```python
from build123d import *

# Parameters (mm, degrees)
SKETCH1_R           = 82.5
BOSS_EXTRUDE1_DEPTH = 17
SKETCH2_R           = 40
CUT_EXTRUDE1_DEPTH  = 118.904622471
SKETCH3_R           = 5.652492576
CUT_EXTRUDE2_DEPTH  = 12.839244
CIRPATTERN1_START   = 4.160755595
CIRPATTERN1_DEPTH   = 12.839244405


# Read off the part's stored shape, not the designer's step: CirPattern1
with BuildPart() as part:
    # Sketch1 → Boss-Extrude1 (new body)
    with BuildSketch(Plane(origin=(0, 0, 0), x_dir=(1, 0, 0), z_dir=(0, 1, 0))):
        with Locations(Location((0, 0, 0), (0, 0, 270))):
            Circle(SKETCH1_R)
    extrude(amount=BOSS_EXTRUDE1_DEPTH)

    # Sketch2 → Cut-Extrude1 (cut, through all)
    with BuildSketch(Plane(origin=(0, 0, 0), x_dir=(1, 0, 0), z_dir=(0, 1, 0))):
        with Locations(Location((0, 0, 0), (0, 0, 270))):
            Circle(SKETCH2_R)
    extrude(amount=CUT_EXTRUDE1_DEPTH, mode=Mode.SUBTRACT)

    # Sketch3 → Cut-Extrude2 (cut)
    with BuildSketch(Plane(origin=(0, 17, 0), x_dir=(1, 0, 0), z_dir=(0, 1, 0))):
        with Locations((-36.098285333, 0)):
            Circle(SKETCH3_R)
    extrude(amount=-CUT_EXTRUDE2_DEPTH, mode=Mode.SUBTRACT)

    # CirPattern1 outline → CirPattern1 (cut)
    with BuildSketch(Plane(origin=(0, 0, 0), x_dir=(1, 0, 0), z_dir=(0, 1, 0)).offset(CIRPATTERN1_START)):
        with BuildLine():
            ThreePointArc((-4.299022975, 39.768309009), (0, 40), (4.299022975, 39.768309009))
            ThreePointArc((4.299022975, 39.768309009), (0, 41.75077791), (-4.299022975, 39.768309009))
        make_face()
        with BuildLine():
            ThreePointArc((39.768309009, -4.299022975), (41.75077791, 0), (39.768309009, 4.299022975))
            ThreePointArc((39.768309009, 4.299022975), (40, 0), (39.768309009, -4.299022975))
        make_face()
        with BuildLine():
            ThreePointArc((4.299022975, -39.768309009), (0, -40), (-4.299022975, -39.768309009))
            ThreePointArc((-4.299022975, -39.768309009), (0, -41.75077791), (4.299022975, -39.768309009))
        make_face()
    extrude(amount=CIRPATTERN1_DEPTH, mode=Mode.SUBTRACT)


solid = part.part
```
Design review of the part built by this model. Coordinates are the model's own, in mm. A direction names the side the tool comes from. Round coordinates to 2 decimals unless told otherwise and drop trailing zeros. Order: outer loops, then holes, each group sorted by start corner. A loop starts at its lowest first (then second) coordinate and runs counter-clockwise, first axis right, second up. Notation, with made-up numbers: M -13.75,15.25 L -3.75,15.25 A32 cw -3.75,54.25 Z; hole C -26,84 d11. An arc over 180 degrees is marked long. Put each result on its own line as item: value.
Q1. Consider section D-D (z = 32). State the section outline as (x, y) points, and give its area (3 significant figures).
Reported:
outline: M -76.04,0 L -24,0 L -24,17 L -76.04,17 Z; M 24,0 L 76.04,0 L 76.04,17 L 24,17 Z
area: 1,770 mm²
Q2. Consider section A-A (z = 0). State the section outline as (x, y) points, and give its area (3 significant figures).
Reported:
outline: M -82.5,0 L -40,0 L -40,4.16 L -41.75,4.16 L -41.75,17 L -82.5,17 Z; M 40,0 L 82.5,0 L 82.5,17 L 41.75,17 L 41.75,4.16 L 40,4.16 Z
area: 1,400 mm²
Q3. To check wall thickness, follow line 1 (Z direction, x = -29.5, y = 5); line 2 (X direction, y = 1.5, z = 14.5); line 3 (Z direction, x = 31, y = 8.5). State the ranges of each line that lie inside material, in increasing order.
Reported:
line 1: -77.05 to -27.01, 27.01 to 77.05
line 2: -81.22 to -37.28, 37.28 to 81.22
line 3: -76.45 to -25.28, 25.28 to 76.45
Q4. Insertion check: pin 1 Ø1 at (x, z) = (-40.5, 0) entering from +Y; pin 2 Ø8 at (y, z) = (7, -54) entering from -X; pin 3 Ø5 at (y, z) = (7.5, -44) entering from -X; pin 4 Ø12 at (x, z) = (18, 34) entering from +Y. Each pin has a flat end and moves straight along its axis. Give the tip position at first contact, or say it passes through.
Reported:
pin 1: y = 4.16
pin 2: x = -65.62
pin 3: x = -71.3
pin 4: y = 17
Q5. Machinability: for faces 4 (the face through (-0.07, 10.49, 41.75)), 5 (the face through (-36, 0, -19)), which of the approach directions +Z, -Z, +X, -X, +Y, -Y give a long, thin tool a straight path to every point of the face, cutting with its end or side? Answer none if there is none.
Reported:
face 4: +Y
face 5: +Z, -Z, +X, -X, -Y
Q6. Consider section C-C (y = 6.5). State the section outline as (x, z) points, and give its area (3 significant figures).
Reported:
outline: C 0,0 d165; hole M -39.77,-4.3 A40 ccw -4.3,-39.77 A5.65 ccw 4.3,-39.77 A40 ccw 39.77,-4.3 A5.65 ccw 39.77,4.3 A40 ccw 4.3,39.77 A5.65 ccw -4.3,39.77 A40 ccw -39.77,4.3 A5.65 ccw Z
area: 16,300 mm²
Q7. Consider section B-B (x = 0). State the section outline as (y, z) points, and give its area (3 significant figures).
Reported:
outline: M 0,-82.5 L 17,-82.5 L 17,-41.75 L 4.16,-41.75 L 4.16,-40 L 0,-40 Z; M 0,40 L 4.16,40 L 4.16,41.75 L 17,41.75 L 17,82.5 L 0,82.5 Z
area: 1,400 mm²
Q8. Draft analysis for pull direction Z (two halves, no side actions). For faces 1 (the face through (-80.54, 8.38, -17.88)), 2 (the face through (-36, 17, -19)), 3 (the face through (-41.75, 10.67, -0.07)), state which applies: released by +Z, released by -Z, zero draft, split by the parting line, or undercut.
Reported:
face 1: split by the parting line
face 2: zero draft
face 3: undercut
